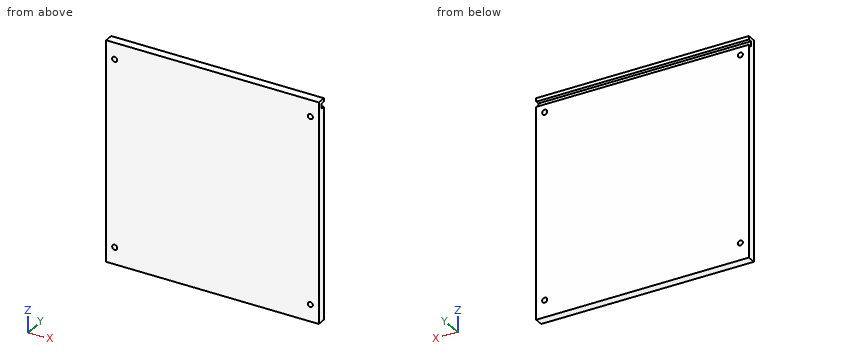
```python
from build123d import *

# Parameters (mm, degrees)
CROQUIS1_W              = 250
CROQUIS1_H              = 260
SALIENTE_EXTRUIR1_DEPTH = 10
CORTAR_EXTRUIR1_REACH   = 252
CROQUIS4_W              = 6.138345694
CROQUIS4_H              = 4.301035896
CORTAR_EXTRUIR2_REACH   = 12
CROQUIS5_R              = 3


with BuildPart() as part:
    # Croquis1 → Saliente-Extruir1 (new body)
    with BuildSketch(Plane(origin=(0, 0, 0), x_dir=(1, 0, 0), z_dir=(0, 1, 0))):
        Rectangle(CROQUIS1_W, CROQUIS1_H)
    extrude(amount=SALIENTE_EXTRUIR1_DEPTH)

    # Croquis4 → Cortar-Extruir1 (cut, up to next)
    with BuildSketch(Plane.ZY.offset(125), mode=Mode.PRIVATE) as cortar_extruir1_sk1:
        with Locations((122.851537289, 7.849482052)):
            Rectangle(CROQUIS4_W, CROQUIS4_H)
    cortar_extruir1_tool1 = extrude(cortar_extruir1_sk1.sketch, amount=-CORTAR_EXTRUIR1_REACH, mode=Mode.PRIVATE) & part.part
    add(cortar_extruir1_tool1.solids().sort_by_distance((-125, 7.849482, 122.851537))[0], mode=Mode.SUBTRACT)

    # Croquis5 → Cortar-Extruir2 (cut, up to next)
    with BuildSketch(Plane.XZ, mode=Mode.PRIVATE) as cortar_extruir2_sk1:
        with Locations((-115, 110.530243228)):
            Circle(CROQUIS5_R)
    cortar_extruir2_tool1 = extrude(cortar_extruir2_sk1.sketch, amount=-CORTAR_EXTRUIR2_REACH, mode=Mode.PRIVATE) & part.part
    add(cortar_extruir2_tool1.solids().sort_by_distance((-115, 0, 110.530243))[0], mode=Mode.SUBTRACT)
    # Croquis5 → Cortar-Extruir2 (cut, up to next)
    with BuildSketch(Plane.XZ, mode=Mode.PRIVATE) as cortar_extruir2_sk2:
        with Locations((115, 110.530243228)):
            Circle(CROQUIS5_R)
    cortar_extruir2_tool2 = extrude(cortar_extruir2_sk2.sketch, amount=-CORTAR_EXTRUIR2_REACH, mode=Mode.PRIVATE) & part.part
    add(cortar_extruir2_tool2.solids().sort_by_distance((115, 0, 110.530243))[0], mode=Mode.SUBTRACT)
    # Croquis5 → Cortar-Extruir2 (cut, up to next)
    with BuildSketch(Plane.XZ, mode=Mode.PRIVATE) as cortar_extruir2_sk3:
        with Locations((-115, -110)):
            Circle(CROQUIS5_R)
    cortar_extruir2_tool3 = extrude(cortar_extruir2_sk3.sketch, amount=-CORTAR_EXTRUIR2_REACH, mode=Mode.PRIVATE) & part.part
    add(cortar_extruir2_tool3.solids().sort_by_distance((-115, 0, -110))[0], mode=Mode.SUBTRACT)
    # Croquis5 → Cortar-Extruir2 (cut, up to next)
    with BuildSketch(Plane.XZ, mode=Mode.PRIVATE) as cortar_extruir2_sk4:
        with Locations((115, -110)):
            Circle(CROQUIS5_R)
    cortar_extruir2_tool4 = extrude(cortar_extruir2_sk4.sketch, amount=-CORTAR_EXTRUIR2_REACH, mode=Mode.PRIVATE) & part.part
    add(cortar_extruir2_tool4.solids().sort_by_distance((115, 0, -110))[0], mode=Mode.SUBTRACT)


solid = part.part
```
CAD build for the part. Positions are in the model's coordinates, mm. Round coordinates to 2 decimals unless told otherwise and drop trailing zeros. Order: outer loops, then holes, each group sorted by start corner. A loop starts at its lowest first (then second) coordinate and runs counter-clockwise, first axis right, second up. Notation, with made-up numbers: (-1.75, 13) -> (14.25, 13) arc R32 ccw to (14.25, 45) -> close; hole circle Ø3 at (-3, 10.25). An arc over 180 degrees is marked (long way). Write item = value, one per line.
(1) Cut at A-A (z = -110). Write the cut outline in (x, y), plus the area to 3 significant figures.
Answers follow:
outline = (-125, 0) -> (-118, 0) -> (-118, 10) -> (-125, 10) -> close; (-112, 0) -> (112, 0) -> (112, 10) -> (-112, 10) -> close; (118, 0) -> (125, 0) -> (125, 10) -> (118, 10) -> close
area = 2,380 mm²
(2) Cut at B-B (x = -115). Write the cut outline in (y, z), plus the area to 3 significant figures.
Answers follow:
outline = (0, -130) -> (10, -130) -> (10, -113) -> (0, -113) -> close; (0, -107) -> (10, -107) -> (10, 107.53) -> (0, 107.53) -> close; (0, 113.53) -> (10, 113.53) -> (10, 119.78) -> (5.7, 119.78) -> (5.7, 125.92) -> (10, 125.92) -> (10, 130) -> (0, 130) -> close
area = 2,450 mm²
(3) Cut at C-C (y = 7.75). Write the cut outline in (x, z).
Answers follow:
outline = (-125, -130) -> (125, -130) -> (125, 119.78) -> (-125, 119.78) -> close; (-125, 125.92) -> (125, 125.92) -> (125, 130) -> (-125, 130) -> close; hole circle Ø6 at (-115, -110); hole circle Ø6 at (-115, 110.53); hole circle Ø6 at (115, -110); hole circle Ø6 at (115, 110.53)
(4) Drill centre lines: L1, parallel to Z at x = -115, y = 4; L2, parallel to Z at x = 55, y = 7.25; L3, parallel to X at y = 4.5, z = -108.5. Where is each one in solid material? Low to high.
Answers follow:
L1 = -130 to -113, -107 to 107.53, 113.53 to 130
L2 = -130 to 119.78, 125.92 to 130
L3 = -125 to -117.6, -112.4 to 112.4, 117.6 to 125
(5) Flat gauge pins, fed straight in: P1, Ø3.5, axis at x = -115, z = -110, coming from the +Y side; P2, Ø1.8, axis at x = -14.5, z = 122, coming from the +Y side. Where does each tip first touch, or does it go through?
Answers follow:
P1 = through
P2 = 5.7
